```python
from build123d import *

# Parameters (mm, degrees)
F1_DEPTH = 10
F0_R     = 17.5
F2_DEPTH = 50
F3_DEPTH = 20


with BuildPart() as f1:
    # F0 (on Front) → F1 (new body)
    with BuildSketch(Plane.XZ):
        with BuildLine():
            Line((27.51959, 20.872951), (-22.48041, 20.872951))
            ThreePointArc((-22.48041, 20.872951), (-40.15808, 13.550621), (-47.48041, -4.127049))
            ThreePointArc((-47.48041, -4.127049), (-40.15808, -21.804718), (-22.48041, -29.127049))
            Line((-22.48041, -29.127049), (27.51959, -29.127049))
            ThreePointArc((27.51959, -29.127049), (2.51959, -4.127049), (27.51959, 20.872951))
        make_face()
    extrude(amount=F1_DEPTH)



with BuildPart() as f2:
    # F0 (on Front) → F2 (new body)
    with BuildSketch(Plane.XZ):
        with Locations((27.51959, -4.127049)):
            Circle(F0_R)
    extrude(amount=F2_DEPTH)


with BuildPart() as f1_1:
    add(f1.part)

    add(f2.part)  # F3 merges F2
    # F0 (on Front) → F3 (join)
    with BuildSketch(Plane.XZ):
        with BuildLine():
            ThreePointArc((52.51959, -4.127049), (45.197259, 13.550621), (27.51959, 20.872951))
            ThreePointArc((27.51959, 20.872951), (2.51959, -4.127049), (27.51959, -29.127049))
            ThreePointArc((27.51959, -29.127049), (45.197259, -21.804718), (52.51959, -4.127049))
        make_face()
        with Locations((27.51959, -4.127049)):
            Circle(F0_R, mode=Mode.SUBTRACT)
    extrude(amount=F3_DEPTH)


solid = f1_1.part
```
The model under review builds one solid part; all positions refer to its coordinate system, in mm. A direction names the side the tool comes from. Coordinates: 2 decimals unless noted, no trailing zeros. Write each loop counter-clockwise with the first axis right and the second up, starting at its lowest first coordinate (ties: lowest second). Pieces come first, ordered by that corner, then holes.
1) We need section C-C on y = -17. State the section outline as (x, z) points.
2) We need section D-D on x = 4. State the section outline as (y, z) points.
3) Machinability: for faces 1 (the face through (27, -50, -4)), 2 (the face through (35.595, -34.79, -19.653)), which of the approach directions +Z, -Z, +X, -X, +Y, -Y give a long, thin tool a straight path to every point of the face, cutting with its end or side? Answer none if there is none.
4) Clearance check with flat-ended pins moving along their axes: pin 1 Ø1 at (x, y) = (18.5, -18.5) entering from -Z; pin 2 Ø6 at (y, z) = (-10, -14.5) entering from +X; pin 3 Ø6 at (y, z) = (-23.5, 14.5) entering from -X. State where each tip first meets the part, or that it passes through.
5) We need section A-A on x = 42.5. State the section outline as (y, z) points.
6) We need section B-B on z = 3. State the section outline as (x, y) points.
7) To check wall thickness, follow probe 1 along Y at (x, z) = (2, -4.5); probe 2 along Z at (x, y) = (28, -38.5); probe 3 along Y at (x, z) = (11, 5). State the ranges of each line that lie inside material, in increasing order.
Answer list:
1. outline: (27.52, -29.13) arc R25 ccw to (52.52, -4.13) arc R25 ccw (long way) to start
2. outline: (-20, -12.6) - (-10, -12.6) - (-10, -29.13) - (0, -29.13) - (0, 20.87) - (-10, 20.87) - (-10, 4.35) - (-20, 4.35) - close
3. face 1: +Z, -Z, +X, -X, -Y
3. face 2: -Y
4. pin 1: stops at z = -27.63
4. pin 2: stops at x = 51.41
4. pin 3: stops at x = 19.64
5. outline: (-50, -13.17) - (-20, -13.17) - (-20, -24.14) - (0, -24.14) - (0, 15.89) - (-20, 15.89) - (-20, 4.92) - (-50, 4.92) - close
6. outline: (-46.44, -10) - (3.56, -10) - (3.56, -20) - (11.54, -20) - (11.54, -50) - (43.5, -50) - (43.5, -20) - (51.48, -20) - (51.48, 0) - (-46.44, 0) - close
7. probe 1: y = -10 to 0
7. probe 2: z = -21.62 to 13.37
7. probe 3: y = -20 to 0
